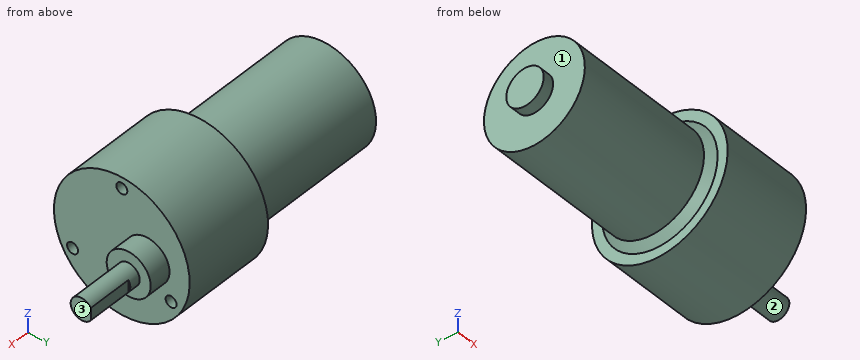
```python
from build123d import *

# Parameters (mm, degrees)
SKETCH_1_R          = 13.75
EXTRUDE_1_DEPTH     = 20
SKETCH_2_R          = 5.1
EXTRUDE_2_DEPTH     = 3
SKETCH_3_R          = 18.5
EXTRUDE_3_DEPTH     = 25
SKETCH_4_R          = 6
EXTRUDE_4_DEPTH     = 6
SKETCH_5_R          = 3
EXTRUDE_5_DEPTH     = 15
CUT_EXTRUDE_1_DEPTH = 12
SKETCH_7_R          = 1.5
CUT_EXTRUDE_2_DEPTH = 3
CHAMFER_1_SIZE      = 2


with BuildPart() as part:
    # ｽｹｯﾁ1 → ﾎﾞｽ - 押し出し1 (new body, symmetric)
    with BuildSketch(Plane(origin=(0, 0, 0), x_dir=(0, 0, -1), z_dir=(1, 0, 0))):
        Circle(SKETCH_1_R)
    extrude(amount=EXTRUDE_1_DEPTH, both=True)

    # ｽｹｯﾁ2 → ﾎﾞｽ - 押し出し2 (add)
    with BuildSketch(Plane.ZY.offset(20)):
        Circle(SKETCH_2_R)
    extrude(amount=EXTRUDE_2_DEPTH)

    # ｽｹｯﾁ3 → ﾎﾞｽ - 押し出し3 (add)
    with BuildSketch(Plane(origin=(20, 0, 0), x_dir=(0, 0, -1), z_dir=(1, 0, 0))):
        Circle(SKETCH_3_R)
    extrude(amount=EXTRUDE_3_DEPTH)

    # ｽｹｯﾁ4 → ﾎﾞｽ - 押し出し4 (add)
    with BuildSketch(Plane(origin=(45, 0, 0), x_dir=(0, 0, -1), z_dir=(1, 0, 0))):
        with Locations((0, 7)):
            Circle(SKETCH_4_R)
    extrude(amount=EXTRUDE_4_DEPTH)

    # ｽｹｯﾁ5 → ﾎﾞｽ - 押し出し5 (add)
    with BuildSketch(Plane(origin=(51, 0, 0), x_dir=(0, 0, -1), z_dir=(1, 0, 0))):
        with Locations((0, 7)):
            Circle(SKETCH_5_R)
    extrude(amount=EXTRUDE_5_DEPTH)

    # ｽｹｯﾁ6 → ｶｯﾄ - 押し出し1 (cut)
    with BuildSketch(Plane(origin=(66, 0, 0), x_dir=(0, 0, -1), z_dir=(1, 0, 0))):
        Polygon((-80.661429966, 9.5), (-1.658312395, 9.5), (1.658312395, 9.5), (80.661429966, 9.5), (80.661429966, 167.506235142), (-80.661429966, 167.506235142), align=None)
    extrude(amount=-CUT_EXTRUDE_1_DEPTH, mode=Mode.SUBTRACT)

    # ｽｹｯﾁ7 → ｶｯﾄ - 押し出し2 (cut)
    with BuildSketch(Plane(origin=(45, 0, 0), x_dir=(0, 0, -1), z_dir=(1, 0, 0))):
        with Locations((-15.5, 0)):
            Circle(SKETCH_7_R)
        with Locations((7.75, 13.423393759)):
            Circle(SKETCH_7_R)
        with Locations((7.75, -13.423393759)):
            Circle(SKETCH_7_R)
    extrude(amount=-CUT_EXTRUDE_2_DEPTH, mode=Mode.SUBTRACT)

    # 面取り1
    chamfer_1_edges = [part.edges().sort_by_distance(p)[0] for p in [
        (20, 0, 13.75),
    ]]
    chamfer(chamfer_1_edges, length=CHAMFER_1_SIZE)


solid = part.part
```
The listing builds one solid part. Answer for the finished solid, in the listing's coordinates (mm). Face numbers are marked on the shaded views. A direction names the side the tool comes from. Give positions to 0.01 mm unless a question says otherwise; leave off trailing zeros. Order: outer loops, then holes, each group sorted by start corner. A loop starts at its lowest first (then second) coordinate and runs counter-clockwise, first axis right, second up.
Item 1: Given pin 1 Ø5 at (y, z) = (10, -13) entering from -X; pin 2 Ø1.5 at (y, z) = (13.5, -7.5) entering from +X; pin 3 Ø11 at (y, z) = (-9, 2) entering from +X, each flat-ended and moving along its own axis, determine where each tip first touches the part or whether it passes through.
From the geometry:
pin 1: stops at x = 18.15
pin 2: stops at x = 42
pin 3: stops at x = 45
Item 2: Find the intervals of material crossed by probe 1 along Y at (x, z) = (43.8, -7.75); probe 2 along X at (y, z) = (-2, 0); probe 3 along X at (y, z) = (3.5, 10), in increasing order.
From the geometry:
probe 1: y = -16.8 to -14.92, -11.92 to 11.92, 14.92 to 16.8
probe 2: x = -23 to 45
probe 3: x = -20 to 45
Item 3: The part is cut by section A-A, the plane z = 0. Give the vertices of the cut face in (x, y).
From the geometry:
outline: (-23, -5.1) - (-20, -5.1) - (-20, -13.75) - (18, -13.75) - (20, -15.75) - (20, -18.5) - (45, -18.5) - (45, 1) - (51, 1) - (51, 4) - (66, 4) - (66, 9.5) - (54, 9.5) - (54, 10) - (51, 10) - (51, 13) - (45, 13) - (45, 18.5) - (20, 18.5) - (20, 15.75) - (18, 13.75) - (-20, 13.75) - (-20, 5.1) - (-23, 5.1) - close
Item 4: Which of the six approach directions +Z, -Z, +X, -X, +Y, -Y give full straight-line access (tool end or side, diameter ignored) to the marked faces 1, 2 and 3?
From the geometry:
face 1: -X
face 2: +X
face 3: +Z, -Z, +X, +Y, -Y
Item 5: The part is cut by section C-C, the plane x = 44. Give the vertices of the cut face in (y, z), and give its area (3 significant figures).
From the geometry:
outline: circle Ø37 at (0, 0); hole circle Ø3 at (-13.42, -7.75); hole circle Ø3 at (0, 15.5); hole circle Ø3 at (13.42, -7.75)
area: 1,050 mm2
Item 6: The part is cut by section B-B, the plane x = 34.5. Give the vertices of the cut face in (y, z).
From the geometry:
outline: circle Ø37 at (0, 0)
Item 7: The part is cut by section D-D, the plane x = -15.5. Give the vertices of the cut face in (y, z).
From the geometry:
outline: circle Ø27.5 at (0, 0)
